Build history of the part. All positions in model axes, mm. A direction names the side the tool comes from. Give positions to 0.01 mm unless a question says otherwise; leave off trailing zeros. Order: outer loops, then holes, each group sorted by start corner. A loop starts at its lowest first (then second) coordinate and runs counter-clockwise, first axis right, second up. Notation, with made-up numbers: (37.25, -25.75) - (76.25, -25.75) arc R19 ccw to (76.25, 3.25) - close; hole circle Ø7 at (17, 12). An arc over 180 degrees is marked (long way). Use a Markdown table: item, result.
Autodesk Inventor part; units mm, degrees
ref_plane "Arbeitsebene1" through (0, 0, 7.5) normal (0, 0, 1) x (1, 0, 0)
ref_plane "YZ Plane" through (0, 0, 0) normal (1, 0, 0) x (0, 1, 0)
ref_plane "XZ Plane" through (0, 0, 0) normal (0, 1, 0) x (-1, 0, 0)
sketch "Skizze1" plane through (0, 0, 0) normal (0, 0, 1) x (1, 0, 0)
  circle A0 centre (0, 0) radius 5
  dimension "d0" = 10
extrude "Extrusion1" add sketch "Skizze1" along normal blind 14
sketch "Skizze2" plane through (0, 0, 0) normal (0, 0, -1) x (-1, 0, 0)
  circle A0 centre (0, 0) radius 4
  dimension "d3" = 8
extrude "Extrusion2" cut sketch "Skizze2" against normal blind 7.5
ref_plane "Arbeitsebene1" through (0, 0, 7.5) normal (0, 0, 1) x (1, 0, 0)
sketch "Skizze3" plane through (0, 0, 7.5) normal (0, 0, 1) x (1, 0, 0)
  point P0 (0, 0)
  point P1 (0, 0)
hole "Bohrung1" at (0, 0, 7.5) direction (0, 0, 1) diameter 1.5 depth 4.5 tip angle 118
chamfer "Fasen1" distance 0.2 angle 45 3 edges at (4, 0, 0) (-5, 0, 0) (-5, 0, 14)
properties part number "Arbeitskolben" material "Bronze, Guss"
1) Two-plate mould, pull along X, no slides. Class faces 1 (the cylindrical face through (-1.08, 4.88, 6.9)), 2 (the flat face through (0, -1, 7.5)), 3 (the flat face through (0, 0, 14)): +X half, -X half, draft (parallel to the pull), parting line (faces both ways), or undercut.
Computed:
| item | result |
|---|---|
| face 1 | parting line |
| face 2 | undercut |
| face 3 | draft |
2) Slice it at B-B (z = 5.5). Write the cut outline in (x, y).
Computed:
| item | result |
|---|---|
| outline | circle Ø10 at (0, 0); hole circle Ø8 at (0, 0) |
3) Tool access for faces 4 (the cylindrical face through (-0.03, -0.75, 9.78)), 5 (the flat face through (2, -4, 0)): list every direction of +Z, -Z, +X, -X, +Y, -Y with a clear straight run to the whole face (end or side of a thin tool).
Computed:
| item | result |
|---|---|
| face 4 | -Z |
| face 5 | -Z, +X, -X, +Y, -Y |
4) Pin check, flat tips, straight feed: P1, Ø1, axis at y = -3, z = 8, coming from the -X side; P2, Ø2, axis at x = 1.5, z = 6.5, coming from the +Y side; P3, Ø4, axis at x = -3, z = 4, coming from the -Y side. Stop position of each tip, or through.
Computed:
| item | result |
|---|---|
| P1 | stops at x = -4.33 |
| P2 | stops at y = 4.97 |
| P3 | stops at y = -4.9 |
5) Slice it at A-A (z = 11.5). Write the cut outline in (x, y).
Computed:
| item | result |
|---|---|
| outline | circle Ø10 at (0, 0); hole circle Ø1.5 at (0, 0) |
6) Wall check: line 1 (Y direction, x = 0, z = 4.5); line 2 (Y direction, x = 0, z = 9.6); line 3 (Z direction, x = 0.5, y = 2.75). Give the ranges that are in metal, low to high. Write a range as from..to.
Computed:
| item | result |
|---|---|
| line 1 | y = -5..-4, 4..5 |
| line 2 | y = -5..-0.75, 0.75..5 |
| line 3 | z = 7.5..14 |
